Check sheet for the modelled part. Datum: model origin and axes. Units: mm. Face numbers are marked on the shaded views. Round coordinates to 2 decimals unless told otherwise and drop trailing zeros. Loops run counter-clockwise (first coordinate to the right, second up) from the corner with the lowest first, then second, coordinate; pieces in that order, holes last. Notation, with made-up numbers: (55, -6.5) -> (75, -6.5) arc R23 cw to (75, 10.5) -> close; hole circle Ø10 at (28, 79.25). An arc over 180 degrees is marked (long way). Use one line per item in the form item = value. Start each with the question number.
(1) Sectioned sample at C-C (x = -12). Record the cut outline in (y, z), and give its area (3 significant figures).
(2) Go/stop test with flat-tipped pins: pin 1 (3.5 mm diameter, centred on x = -25, z = 11, fed in from +Y); pin 2 (6 mm diameter, centred on x = 6, y = 33, fed in from +Z); pin 3 (5 mm diameter, centred on x = 25, z = 11, fed in from -Y). Record where each tip stops, or that it passes through.
(3) Sectioned sample at D-D (z = 1.25). Record the cut outline in (x, y), and give its area (3 significant figures).
(4) Draft check along Y on the marked faces 1, 2 and 3. Enter one of: released by +Y, released by -Y, zero draft, split by the parting line, or undercut.
(5) Sectioned sample at B-B (x = 0). Record the cut outline in (y, z).
(6) Material ranges on probe 1 along X at (y, z) = (112.5, 11); probe 2 along Y at (x, z) = (-3.5, 4.25); probe 3 along Y at (x, z) = (1, 14.75), recorded low to high. Write a range as [from, to].
(7) Sectioned sample at A-A (y = 0). Record the cut outline in (x, z), and give its area (3 significant figures).
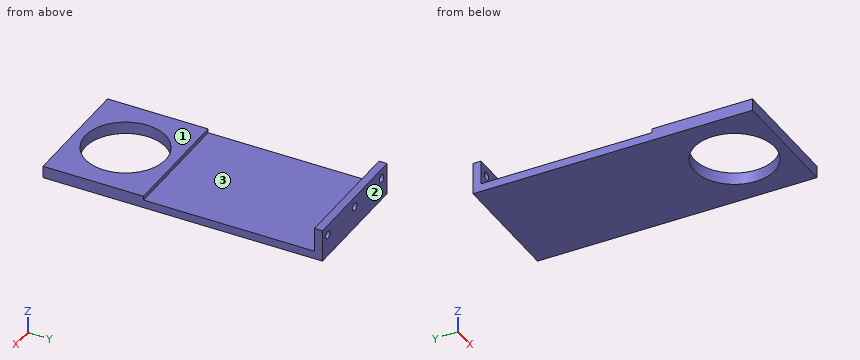
from build123d import *

# Parameters (mm, degrees)
SKETCH1_W           = 60
SKETCH1_H           = 50
SKETCH1_R           = 20
BOSS_EXTRUDE1_DEPTH = 6
SKETCH1_3_W         = 60
SKETCH1_3_H         = 85
BOSS_EXTRUDE2_DEPTH = 4
SKETCH4_W           = 60
SKETCH4_H           = 16
SKETCH4_R           = 2
BOSS_EXTRUDE3_DEPTH = 4


with BuildPart() as part:
    # Sketch1 → Boss-Extrude1 (new body)
    with BuildSketch(Plane.XY):
        Rectangle(SKETCH1_W, SKETCH1_H)
        Circle(SKETCH1_R, mode=Mode.SUBTRACT)
    extrude(amount=BOSS_EXTRUDE1_DEPTH)

    # Sketch1_3 → Boss-Extrude2 (add)
    with BuildSketch(Plane.XY):
        with Locations((0, 67.5)):
            Rectangle(SKETCH1_3_W, SKETCH1_3_H)
    extrude(amount=BOSS_EXTRUDE2_DEPTH)

    # Sketch4 → Boss-Extrude3 (add)
    with BuildSketch(Plane(origin=(0, 110, 0), x_dir=(1, 0, 0), z_dir=(0, 1, 0))):
        with Locations((0, -8)):
            Rectangle(SKETCH4_W, SKETCH4_H)
        with Locations(Location((-25, -11, 0), (0, 0, 270))):
            Circle(SKETCH4_R, mode=Mode.SUBTRACT)
        with Locations(Location((0, -11, 0), (0, 0, 270))):
            Circle(SKETCH4_R, mode=Mode.SUBTRACT)
        with Locations(Location((25, -11, 0), (0, 0, 270))):
            Circle(SKETCH4_R, mode=Mode.SUBTRACT)
    extrude(amount=BOSS_EXTRUDE3_DEPTH)


solid = part.part
Checks:
q1.outline = (-25, 0) -> (-16, 0) -> (-16, 6) -> (-25, 6) -> close; (16, 0) -> (114, 0) -> (114, 16) -> (110, 16) -> (110, 4) -> (25, 4) -> (25, 6) -> (16, 6) -> close
q1.area = 512 mm2
q2.pin_1 = through
q2.pin_2 = 4
q2.pin_3 = 110
q3.outline = (-30, -25) -> (30, -25) -> (30, 114) -> (-30, 114) -> close; hole circle Ø40 at (0, 0)
q3.area = 7,080 mm2
q4.face_1 = zero draft
q4.face_2 = released by +Y
q4.face_3 = undercut
q5.outline = (-25, 0) -> (-20, 0) -> (-20, 6) -> (-25, 6) -> close; (20, 0) -> (114, 0) -> (114, 9) -> (110, 9) -> (110, 4) -> (25, 4) -> (25, 6) -> (20, 6) -> close; (110, 13) -> (114, 13) -> (114, 16) -> (110, 16) -> close
q6.probe_1 = [-30, -27], [-23, -2], [2, 23], [27, 30]
q6.probe_2 = [-25, -19.69], [19.69, 25], [110, 114]
q6.probe_3 = [110, 114]
q7.outline = (-30, 0) -> (-20, 0) -> (-20, 6) -> (-30, 6) -> close; (20, 0) -> (30, 0) -> (30, 6) -> (20, 6) -> close
q7.area = 120 mm2
